Autodesk Inventor part; units mm, degrees
ref_plane "FDT_MOUNT_XY" through (0, -10.7, 0) normal (0, 1, 0) x (-1, 0, 0)
ref_plane "FDT_MOUNT_YZ" through (0, -10.7, 0) normal (-1, 0, 0) x (0, 0, 1)
ref_plane "FDT_MOUNT_ZX" through (0, -10.7, 0) normal (0, 0, 1) x (0, 1, 0)
sketch "Sketch_6" plane through (0, 0, 0) normal (0, 0, 1) x (1, 0, 0)
  line L0 (0, -14.05) -> (0, 10.1)
  line L1 (0, 10.1) -> (1.2, 10.1)
  line L2 (1.2, 10.1) -> (2.1, 8.9)
  line L3 (2.1, 8.9) -> (2.1, 9.7)
  line L4 (2.1, 9.7) -> (2.2865, 10.1)
  line L5 (2.2865, 10.1) -> (2.4, 10.1)
  line L6 (2.4, 10.1) -> (2.6, 9.9)
  line L7 (2.6, 9.9) -> (2.6, 8.9)
  line L8 (2.6, 8.9) -> (3.75, 8.9)
  line L9 (3.75, 8.9) -> (4.45, 8.4959)
  line L10 (4.45, 8.4959) -> (4.45, 4.15)
  line L11 (4.45, 4.15) -> (3.75, 4.15)
  line L12 (3.75, 4.15) -> (3.75, 4.1)
  line L13 (3.75, 4.1) -> (4.45, 4.1)
  line L14 (4.45, 4.1) -> (4.45, -9.65)
  line L15 (4.45, -9.65) -> (3.7264, -9.65)
  arc A0 (3.7264, -9.65) -> (3.95, -9.75) centre (3.95, -9.45) ccw
  line L16 (3.95, -9.75) -> (4.2, -9.75)
  line L17 (4.2, -9.75) -> (4.2, -10.45)
  line L18 (4.2, -10.45) -> (3.9, -10.45)
  line L19 (3.9, -10.45) -> (3.9, -10.7)
  line L20 (3.9, -10.7) -> (2.5, -10.7)
  line L21 (2.5, -10.7) -> (2.5, -13.5595)
  line L22 (2.5, -13.5595) -> (2.0095, -14.05)
  line L23 (2.0095, -14.05) -> (0, -14.05)
  line L24 (0, -14.05) -> (0, 10.1)
revolve "Revolution1" add sketch "Sketch_6" angle 360 about axis through (0, -14.05, 0) along (0, -1, 0)
thread "Thread1"
sketch "Sketch_8" plane through (0, 10.1, 0) normal (0, 1, 0) x (1, 0, 0)
  line L0 (-0.3, 1.9774) -> (-0.3, -1.9774)
  arc A0 (-0.3, -1.9774) -> (0.3, -1.9774) centre (0, 0) ccw
  line L1 (0.3, -1.9774) -> (0.3, 1.9774)
  arc A1 (0.3, 1.9774) -> (-0.3, 1.9774) centre (0, 0) ccw
extrude "Extrusion1" cut sketch "Sketch_8" against normal blind 1
sketch "Sketch_15" plane through (0, 10.1, 0) normal (0, 1, 0) x (1, 0, 0)
  line L0 (-8, -4.6188) -> (0, -9.2376)
  line L1 (0, -9.2376) -> (8, -4.6188)
  line L2 (8, -4.6188) -> (8, 4.6188)
  line L3 (8, 4.6188) -> (0, 9.2376)
  line L4 (0, 9.2376) -> (-8, 4.6188)
  line L5 (-8, 4.6188) -> (-8, -4.6188)
  line L6 (-4, -2.3094) -> (0, -4.6188)
  line L7 (0, -4.6188) -> (4, -2.3094)
  line L8 (4, -2.3094) -> (4, 2.3094)
  line L9 (4, 2.3094) -> (0, 4.6188)
  line L10 (0, 4.6188) -> (-4, 2.3094)
  line L11 (-4, 2.3094) -> (-4, -2.3094)
extrude "Extrusion2" cut sketch "Sketch_15" against normal blind 4.75
sketch "Sketch_11" plane through (0, 0, 0) normal (1, 0, 0) x (0, 1, 0)
  line L0 (0, 0) -> (0, 20.3)
  line L1 (0, 20.3) -> (2.3, 20.3)
  line L2 (2.3, 20.3) -> (4.7847, 19.8619)
  arc A0 (4.95, 19.6649) -> (4.7847, 19.8619) centre (4.75, 19.6649) ccw
  line L3 (4.95, 19.6649) -> (4.95, 18.8)
  line L4 (4.95, 18.8) -> (3.1, 18.8)
  arc A1 (3.1, 18.8) -> (2.7, 18.4) centre (3.1, 18.4) ccw
  line L5 (2.7, 18.4) -> (2.7, 17.8)
  line L6 (2.7, 17.8) -> (3.55, 17.8)
  line L7 (3.55, 17.8) -> (3.75, 17.6)
  line L8 (3.75, 17.6) -> (3.75, 16.4)
  line L9 (3.75, 16.4) -> (4.85, 16.4)
  line L10 (4.85, 16.4) -> (4.85, 14.9)
  line L11 (4.85, 14.9) -> (5, 14.6402)
  line L12 (5, 14.6402) -> (5, 6.85)
  line L13 (5, 6.85) -> (3.6, 5.45)
  line L14 (3.6, 5.45) -> (3.6, 0)
  line L15 (3.6, 0) -> (0, 0)
  line L16 (0, 0) -> (0, 20.3)
revolve "Revolution2" add sketch "Sketch_11" angle 360 about axis through (0, 0, 0) along (0, 0, -1)
sketch "Sketch_10" plane through (0, 0, 0) normal (0, 0, 1) x (1, 0, 0)
  line L0 (-9.8, 34.2) -> (-9.8, -25.8)
  line L1 (-9.8, -25.8) -> (9.8, -25.8)
  line L2 (9.8, -25.8) -> (9.8, 34.2)
  line L3 (9.8, 34.2) -> (-9.8, 34.2)
  line L4 (-4.9, 29.2) -> (-4.9, -20.8)
  line L5 (-4.9, -20.8) -> (4.9, -20.8)
  line L6 (4.9, -20.8) -> (4.9, 29.2)
  line L7 (4.9, 29.2) -> (-4.9, 29.2)
extrude "Extrusion3" cut sketch "Sketch_10" along normal blind 18.3
sketch "Sketch_5" plane through (0, 0, 0) normal (1, 0, 0) x (0, 1, 0)
  line L0 (0, 0) -> (0, 20.3)
  line L1 (0, 20.3) -> (2.3, 20.3)
  arc A0 (2.3, 20.3) -> (2, 20) centre (2.3, 20) ccw
  line L2 (2, 20) -> (2, 5.3)
  line L3 (2, 5.3) -> (1, 5.3)
  line L4 (1, 5.3) -> (1, 0)
  line L5 (1, 0) -> (0, 0)
  line L6 (0, 0) -> (0, 20.3)
revolve "Revolution3" cut sketch "Sketch_5" angle 360 about axis through (0, 0, 0) along (0, 0, -1)
sketch "Sketch7" plane through (0, -14.05, 0) normal (0, -1, 0) x (1, 0, 0)
  point P0 (0, 0)
hole "Hole1" at (0, -14.05, 0) direction (0, 1, 0) diameter 2 depth 16.05 countersink diameter 2.3464 countersink angle 60
ref_plane "FDT_MOUNT_XY" through (0, -10.7, 0) normal (0, 1, 0) x (-1, 0, 0)
ref_plane "FDT_MOUNT_YZ" through (0, -10.7, 0) normal (-1, 0, 0) x (0, 0, 1)
ref_plane "FDT_MOUNT_ZX" through (0, -10.7, 0) normal (0, 0, 1) x (0, 1, 0)
ref_plane "FDT_SCHLAUCH_XY" through (0, 0, 5.3) normal (0, 0, 1) x (1, 0, 0)
ref_plane "FDT_SCHLAUCH_YZ" through (0, 0, 5.3) normal (1, 0, 0) x (0, 1, 0)
ref_plane "FDT_SCHLAUCH_ZX" through (0, 0, 5.3) normal (0, 1, 0) x (0, 0, 1)
ref_plane "Zylinder_XY" through (0, -14.05, 0) normal (0, 1, 0) x (1, 0, 0)
ref_plane "Zylinder_YZ" through (0, -14.05, 0) normal (1, 0, 0) x (0, 0, -1)
ref_plane "Zylinder_ZX" through (0, -14.05, 0) normal (0, 0, -1) x (0, 1, 0)
ref_plane "anbau_XY" through (0, -10.7, 0) normal (0, 1, 0) x (1, 0, 0)
ref_plane "anbau_YZ" through (0, -10.7, 0) normal (1, 0, 0) x (0, 0, -1)
ref_plane "anbau_ZX" through (0, -10.7, 0) normal (0, 0, -1) x (0, 1, 0)
properties part number "193138 GRLA-M5-QS-4-D"
Work out the finished part from the listing and answer in its coordinate system (mm). A direction names the side the tool comes from. Coordinates: 2 decimals unless noted, no trailing zeros. Write each loop counter-clockwise with the first axis right and the second up, starting at its lowest first coordinate (ties: lowest second). Pieces come first, ordered by that corner, then holes. Notation, with made-up numbers: M 15,52 L 68,52 A21 ccw 68,77 Z; hole C 15,-2.75 d1. An arc over 180 degrees is marked long. Use one line per item in the form item = value. Start each with the question number.
1. A tool of negligible diameter and unlimited length cuts with its end or side. For faces 1 (the face through (1.976, 7.077, 3.478)), 2 (the face through (3, -1, 17.8)), 3 (the face through (-1.976, 7.077, -3.478)), from which of +Z, -Z, +X, -X, +Y, -Y can it reach the whole face along a straight path? Write none if from no direction.
2. The mould has two halves that part along Z. Classify faces 4 (the face through (-2, 0, 13)), 5 (the face through (0.63, 9.89, -1.2)), 6 (the face through (-2.636, -0.585, 18.096)), 7 (the face through (-1, 1, 5.3)): released by +Z, released by -Z, zero draft, split by the parting line, or undercut.
3. The part is cut by section A-A (y = 8). Give the vertices of the cut face in (x, z), plus the area to 3 significant figures.
4. Straight lines are drawn through the part: probe 1 along Z at (x, y) = (0, 9.4); probe 2 along X at (y, z) = (0, 11); probe 3 along X at (y, z) = (0, 2.45). For each, find the intervals that lie inside material, in ascending order. Write a range as from..to.
5. The part is cut by section B-B (z = 7.5). Give the vertices of the cut face in (x, y), plus the area to 3 significant figures.
6. Each of these flat-tipped pins is pushed along its axis until it touches: P1, Ø1, axis at x = -3, z = 3.5, coming from the +Y side; P2, Ø4, axis at y = 5.5, z = 8.5, coming from the -X side; P3, Ø3, axis at x = 1, y = -8, coming from the +Z side. Where does it stop, or does it pass through?
7. The part is cut by section C-C (y = -7.5). Give the vertices of the cut face in (x, z).
Evaluation:
q1.face_1 = +Z, +X, +Y
q1.face_2 = none
q1.face_3 = -Z, -X, +Y
q2.face_4 = zero draft
q2.face_5 = undercut
q2.face_6 = undercut
q2.face_7 = released by +Z
q3.outline = M -4,-1.95 A4.45 ccw -3.69,-2.49 L -0.31,-4.44 A4.45 ccw 0.31,-4.44 L 3.69,-2.49 A4.45 ccw 4,-1.95 L 4,1.95 A4.45 ccw 3.69,2.49 L 0.31,4.44 A4.45 ccw -0.31,4.44 L -3.69,2.49 A4.45 ccw -4,1.95 Z
q3.area = 55.1 mm^2
q4.probe_1 = -2.6..-2.1, 2.1..2.6
q4.probe_2 = -4.9..-2, 2..4.9
q4.probe_3 = -3.71..-1, 1..3.71
q5.outline = M -4.9,-0.99 A5 ccw 4.9,-0.99 L 4.9,0.99 A5 ccw -4.9,0.99 Z; hole C 0,0 d4
q5.area = 65.7 mm^2
q6.P1 = 5.35
q6.P2 = -3.57
q6.P3 = 4.45
q7.outline = C 0,0 d8.9; hole C 0,0 d2
